Could you check a few things on this model? Use its own coordinates, in mm. A direction names the side the tool comes from. Round coordinates to 2 decimals unless told otherwise and drop trailing zeros. Order: outer loops, then holes, each group sorted by start corner. A loop starts at its lowest first (then second) coordinate and runs counter-clockwise, first axis right, second up.
```python
from build123d import *

# Parameters (mm, degrees)
F0_R     = 2.5
F1_DEPTH = 3.5
F2_DEPTH = 2
F4_DEPTH = 3
F6_D     = 3
F8_DEPTH = 1


with BuildPart() as f1:
    # F0 (on Front) → F1 (new body, symmetric)
    with BuildSketch(Plane.XZ):
        with BuildLine():
            Line((-15.9480972197, 5), (-16.6897546064, 5))
            Line((-16.6897546064, 5), (-16.6897546064, 0))
            Line((-16.6897546064, 0), (-15.9480972197, 0))
            ThreePointArc((-15.9480972197, 0), (-15.3835115664, 1.1937569599), (-15.1897546064, 2.5))
            ThreePointArc((-15.1897546064, 2.5), (-15.3835115664, 3.8062430401), (-15.9480972197, 5))
        make_face()
        with BuildLine():
            Line((-16.6897546064, 0), (-16.6897546064, 5))
            Line((-16.6897546064, 5), (-15.9480972197, 5))
            ThreePointArc((-15.9480972197, 5), (-24.1897546064, 2.5), (-15.9480972197, 0))
            Line((-15.9480972197, 0), (-16.6897546064, 0))
        make_face()
        with Locations((-19.6897546064, 2.5)):
            Circle(F0_R, mode=Mode.SUBTRACT)
    extrude(amount=F1_DEPTH, both=True)

    # F0 (on Front) → F2 (join, symmetric)
    with BuildSketch(Plane.XZ):
        with BuildLine():
            Line((-16.6897546064, 0), (-16.6897546064, 5))
            Line((-16.6897546064, 5), (-15.9480972197, 5))
            ThreePointArc((-15.9480972197, 5), (-24.1897546064, 2.5), (-15.9480972197, 0))
            Line((-15.9480972197, 0), (-16.6897546064, 0))
        make_face()
        with Locations((-19.6897546064, 2.5)):
            Circle(F0_R, mode=Mode.SUBTRACT)
        with BuildLine():
            Line((-15.9480972197, 5), (-16.6897546064, 5))
            Line((-16.6897546064, 5), (-16.6897546064, 0))
            Line((-16.6897546064, 0), (-15.9480972197, 0))
            ThreePointArc((-15.9480972197, 0), (-15.3835115664, 1.1937569599), (-15.1897546064, 2.5))
            ThreePointArc((-15.1897546064, 2.5), (-15.3835115664, 3.8062430401), (-15.9480972197, 5))
        make_face()
        with BuildLine():
            Line((5.3102453936, 5), (-15.9480972197, 5))
            ThreePointArc((-15.9480972197, 5), (-15.3835115664, 3.8062430401), (-15.1897546064, 2.5))
            ThreePointArc((-15.1897546064, 2.5), (-15.3835115664, 1.1937569599), (-15.9480972197, 0))
            Line((-15.9480972197, 0), (2.3102453936, 0))
            Line((2.3102453936, 0), (2.3102453936, -15))
            Line((2.3102453936, -15), (5.3102453936, -15))
            Line((5.3102453936, -15), (5.3102453936, 5))
        make_face()
    extrude(amount=F2_DEPTH, both=True)

    # F3 (on face) → F4 (join)
    with BuildSketch(Plane(origin=(2.3102453936, 0, 0), x_dir=(0, -1, 0), z_dir=(-1, 0, 0))):
        with BuildLine():
            ThreePointArc((-2, -9.5358983849), (-2, -16.4641016151), (4, -13))
            ThreePointArc((4, -13), (3.4641016151, -11), (2, -9.5358983849))
            Line((2, -9.5358983849), (2, -15))
            Line((2, -15), (-2, -15))
            Line((-2, -15), (-2, -9.5358983849))
        make_face()
        with BuildLine():
            Line((2, -15), (2, -9.5358983849))
            ThreePointArc((2, -9.5358983849), (0, -9), (-2, -9.5358983849))
            Line((-2, -9.5358983849), (-2, -15))
            Line((-2, -15), (2, -15))
        make_face()
    extrude(amount=-F4_DEPTH)

    # F6 (through all)
    with Locations(Plane(origin=(2.3102453936, 0, 0), x_dir=(0, -1, 0), z_dir=(-1, 0, 0))):
        with Locations((0, -13)):
            Hole(F6_D / 2)

    # F7 (on Front) → F8 (join, symmetric)
    with BuildSketch(Plane.XZ):
        Polygon((2.3102453936, 0), (-11.6897546064, 0), (2.3102453936, -8), align=None)
    extrude(amount=F8_DEPTH, both=True)


solid = f1.part
```
Q1. Imagine slicing it at C-C, the plane x = -0.5. Please give me the cut outline in (y, z), then the cut area to 3 significant figures.
Q2. Imagine slicing it at D-D, the plane z = -8.5. Please give me the cut outline in (x, y), then the cut area to 3 significant figures.
Q3. For faces 1 (the flat face through (-2, -1, -2)), 2 (the flat face through (-5, 0, 5)), 3 (the flat face through (-4.788, -0.014, -3.944)), which set-ups out of +Z, -Z, +X, -X, +Y, -Y let a thin tool reach every point of the face, with its end or its side?
Q4. Imagine slicing it at A-A, the plane y = 0. Please give me the cut outline in (x, z), then the cut area to 3 significant figures.
Q5. Imagine slicing it at B-B, the plane z = 2.5. Please give me the cut outline in (x, y).
Q6. We'd pull the mould along X, two halves only. Please class faces 4 (the flat face through (-9, -1.4, 0)), 5 (the flat face through (-3, 2, 1)), 6 (the flat face through (-2, 1, -2)), 7 (the flat face through (5.31, 0, -6)): released by +X, released by -X, zero draft, split by the parting line, or undercut.
Q7. I need wall thicknesses on L1, parallel to Z at x = 3.4, y = 0; L2, parallel to X at y = 1.5, z = -4.75; L3, parallel to X at y = 0.5, z = -1.5. Which ranges of each line are inside material? Lowest first, please.
Q8. For P1, Ø1.2, axis at x = -1.5, y = 0, coming from the +Z side; P2, Ø10, axis at x = -20.5, z = 3, coming from the -Y side; P3, Ø1, axis at x = -18, y = -1.5, coming from the -Z side; P4, Ø2.5, axis at x = -8, z = -4, coming from the -Y side, each with a flat end and sliding along its axis, tell me the tip position at first contact or that it passes through.
Filled in:
1. outline: (-2, 0) - (-1, 0) - (-1, -6.39) - (1, -6.39) - (1, 0) - (2, 0) - (2, 5) - (-2, 5) - close
1. area: 32.8 mm2
2. outline: (2.31, -2) - (5.31, -2) - (5.31, 2) - (2.31, 2) - close
2. area: 12.0 mm2
3. face 1: -Z, -Y
3. face 2: +Z, +X, +Y, -Y
3. face 3: -Z, +Y, -Y
4. outline: (-15.95, 0) - (-11.69, 0) - (2.31, -8) - (2.31, -11.5) - (5.31, -11.5) - (5.31, 5) - (-15.95, 5) arc R4.5 ccw (long way) to start; (2.31, -17) - (5.31, -17) - (5.31, -14.5) - (2.31, -14.5) - close; hole circle Ø5 at (-19.69, 2.5)
4. area: 246 mm2
5. outline: (-24.19, -3.5) - (-22.19, -3.5) - (-22.19, 3.5) - (-24.19, 3.5) - close; (-17.19, -3.5) - (-15.19, -3.5) - (-15.19, -2) - (5.31, -2) - (5.31, 2) - (-15.19, 2) - (-15.19, 3.5) - (-17.19, 3.5) - close
6. face 4: undercut
6. face 5: zero draft
6. face 6: undercut
6. face 7: released by +X
7. L1: z = -17 to -14.5, -11.5 to 5
7. L2: x = 2.31 to 5.31
7. L3: x = -21.75 to -17.63, -9.06 to 5.31
8. P1: stops at z = 5
8. P2: stops at y = -3.5
8. P3: stops at z = -1.84
8. P4: passes through
